Autodesk Inventor part; units mm, degrees
ref_plane "YZ Plane" through (0, 0, 0) normal (1, 0, 0) x (0, 1, 0)
ref_plane "XZ Plane" through (0, 0, 0) normal (0, 1, 0) x (-1, 0, 0)
ref_plane "XY Plane" through (0, 0, 0) normal (0, 0, 1) x (1, 0, 0)
sketch "Sketch1" plane through (0, 0, 0) normal (0, 0, 1) x (1, 0, 0)
  line L0 (-37.1, -32.05) -> (37.1, -32.05)
  line L1 (37.1, 32.05) -> (-37.1, 32.05)
  circle A0 centre (0, 0) radius 25.4
  line L2 (37.1, -32.05) -> (37.1, 32.05)
  line L3 (-37.1, 32.05) -> (-37.1, -32.05)
  dimension "d0" = 50.8
extrude "Lens body" add sketch "Sketch1" along normal blind 12.7 contours A0
sketch "Sketch2" plane through (0, 0, 12.7) normal (0, 0, 1) x (1, 0, 0)
  circle A0 centre (0, 0) radius 25.4
  circle A1 centre (0, 0) radius 12.7
  dimension "d3" = 25.4
extrude "Ring" add sketch "Sketch2" along normal blind 6.35 contours A1
sketch "Sketch5" plane through (0, 0, 19.05) normal (0, 0, 1) x (1, 0, 0)
  circle A0 centre (0, 0) radius 12.7
  circle A1 centre (0, 0) radius 10.16
  dimension "d14" = 2.54
extrude "Pit" cut sketch "Sketch5" against normal blind 6.35 contours A1
sketch "Sketch6" plane through (0, 0, 12.7) normal (0, 0, 1) x (1, 0, 0)
  line L0 (4.445, 6.35) -> (-4.445, 6.35)
  line L1 (-4.445, 6.35) -> (-4.445, -6.35)
  line L2 (-4.445, -6.35) -> (4.445, -6.35)
  line L3 (4.445, -6.35) -> (4.445, 6.35)
  line L4 (4.445, 6.35) -> (-4.445, -6.35) construction
  line L5 (-4.445, 6.35) -> (4.445, -6.35) construction
  point P0 (0, 0)
  dimension "d17" = 12.7
  dimension "d18" = 8.89
extrude "Shutters" cut sketch "Sketch6" against normal blind 1
sketch "Sketch7" plane through (0, 0, 11.7) normal (0, 0, 1) x (1, 0, 0)
  line L0 (-4.445, 6.35) -> (4.445, 6.35)
  line L1 (-4.445, -6.35) -> (-4.445, 6.35)
  line L2 (4.445, -6.35) -> (-4.445, -6.35)
  line L3 (4.445, 6.35) -> (4.445, -6.35)
  line L4 (4.445, -6.35) -> (-4.445, -6.35)
  line L5 (-0.25, 6.35) -> (0.25, 6.35)
  line L6 (0.25, 6.35) -> (0.25, -6.35)
  line L7 (0.25, -6.35) -> (-0.25, -6.35)
  line L8 (-0.25, -6.35) -> (-0.25, 6.35)
  line L9 (-0.25, 6.35) -> (0.25, -6.35) construction
  line L10 (0.25, 6.35) -> (-0.25, -6.35) construction
  point P0 (0, 0)
  dimension "d21" = 0.5
extrude "Extrusion7" cut sketch "Sketch7" against normal blind 0.5 contours L0 L6 L2 L8
properties part number "Lens"
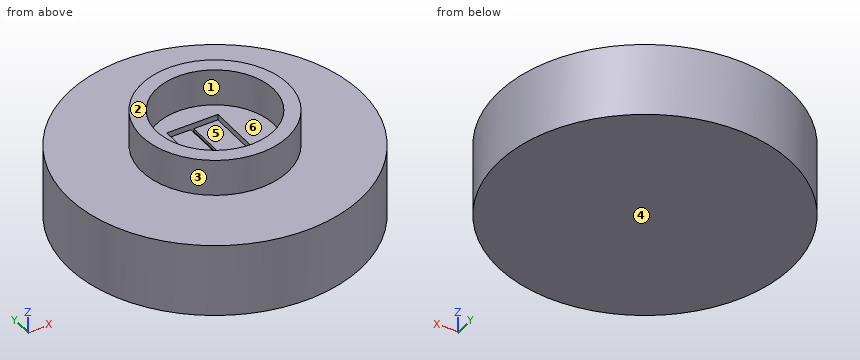
Source: CAD feature listing. Evaluate the final solid. Frame: model axes, mm. Face numbers are marked on the shaded views. A direction names the side the tool comes from. Round coordinates to 2 decimals unless told otherwise and drop trailing zeros. Order: outer loops, then holes, each group sorted by start corner. A loop starts at its lowest first (then second) coordinate and runs counter-clockwise, first axis right, second up. Notation, with made-up numbers: (-39, 74.25) - (-19, 74.25) arc R15 ccw to (-19, 87.25) - close; hole circle Ø2 at (20.25, -38.5). An arc over 180 degrees is marked (long way). Use a Markdown table: item, result. Add a question column.
1. First-contact query: pin 1 (0.5 mm diameter, centred on y = -0.5, z = 12, fed in from -X); pin 2 (2 mm diameter, centred on x = -9.5, y = -17, fed in from +Z); pin 3 (1.5 mm diameter, centred on x = -11.5, z = 15, fed in from -Y). Flat tips, straight axial feed; report the tip coordinate or a pass-through.
2. Section query A-A (y = 0). Return the cut outline in (x, z) (3 decimals).
3. Line query: probe 1 along Y at (x, z) = (0, 16); probe 2 along X at (y, z) = (-9, 16.5); probe 3 along Z at (x, y) = (16, 13). Output: solid intervals per line, ascending.
4. Section query B-B (z = 1.5). Return the cut outline in (x, y), then the cut area to 3 significant figures.
5. Section query D-D (y = -7.5). Return the cut outline in (x, z), then the cut area to 3 significant figures.
6. Set-up query: the marked faces 1 and 2. Return all of +Z, -Z, +X, -X, +Y, -Y with unobstructed straight access to the full face (end or side cutting, diameter ignored); none if empty.
7. Section query C-C (z = 17). Return the cut outline in (x, y).
8. Mould query, pull axis Y, two halves, no side actions, for the marked faces 3, 4, 5 and 6. Classes: +Y half, -Y half, draft (parallel to the pull), parting line (faces both ways), or undercut.
Derived:
| question | item | result |
|---|---|---|
| 1 | pin 1 | x = -25.4 |
| 1 | pin 2 | z = 12.7 |
| 1 | pin 3 | y = -6.76 |
| 2 | outline | (-25.4, 0) - (25.4, 0) - (25.4, 12.7) - (12.7, 12.7) - (12.7, 19.05) - (10.16, 19.05) - (10.16, 12.7) - (4.445, 12.7) - (4.445, 11.7) - (0.25, 11.7) - (0.25, 11.2) - (-0.25, 11.2) - (-0.25, 11.7) - (-4.445, 11.7) - (-4.445, 12.7) - (-10.16, 12.7) - (-10.16, 19.05) - (-12.7, 19.05) - (-12.7, 12.7) - (-25.4, 12.7) - close |
| 3 | probe 1 | -12.7 to -10.16, 10.16 to 12.7 |
| 3 | probe 2 | -8.96 to -4.71, 4.71 to 8.96 |
| 3 | probe 3 | 0 to 12.7 |
| 4 | outline | circle Ø50.8 at (0, 0) |
| 4 | area | 2,030 mm2 |
| 5 | outline | (-24.27, 0) - (24.27, 0) - (24.27, 12.7) - (10.25, 12.7) - (10.25, 19.05) - (6.85, 19.05) - (6.85, 12.7) - (-6.85, 12.7) - (-6.85, 19.05) - (-10.25, 19.05) - (-10.25, 12.7) - (-24.27, 12.7) - close |
| 5 | area | 660 mm2 |
| 6 | face 1 | +Z |
| 6 | face 2 | +Z, +X, -X, +Y, -Y |
| 7 | outline | circle Ø25.4 at (0, 0); hole circle Ø20.32 at (0, 0) |
| 8 | face 3 | parting line |
| 8 | face 4 | draft |
| 8 | face 5 | undercut |
| 8 | face 6 | undercut |
